Here's how the part is built. I have some questions about the finished solid (model axes, mm). Give positions to 0.01 mm unless a question says otherwise; leave off trailing zeros. Loops run counter-clockwise (first coordinate to the right, second up) from the corner with the lowest first, then second, coordinate; pieces in that order, holes last.
Q1. I need wall thicknesses on line 1 (Z direction, x = -27.5, y = 53); line 2 (Z direction, x = -27.65, y = 38.5); line 3 (Y direction, x = -26.05, z = 37.75). Which ranges of each line are inside material? Lowest first, please.
Q2. If we section it at B-B (y = 37): Please give me the cut outline in (x, z).
Q3. If we section it at A-A (z = 36.5): Please give me the cut outline in (x, y).
Q4. If we section it at C-C (x = -26.85): Please give me the cut outline in (y, z).
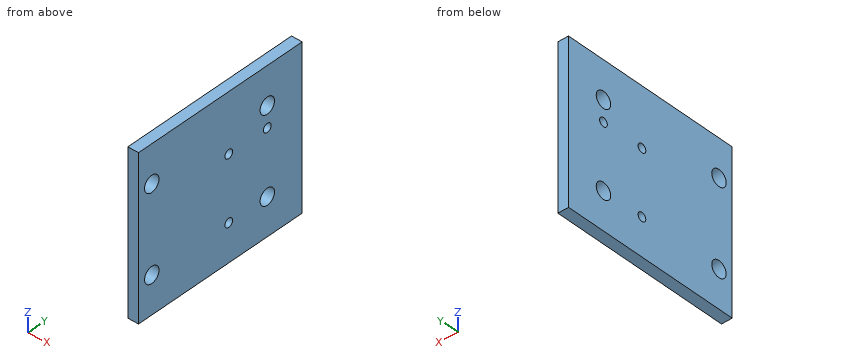
Autodesk Inventor part; units mm, degrees
ref_plane "YZ Plane" through (0, 0, 0) normal (1, 0, 0) x (0, 1, 0)
ref_plane "XZ Plane" through (0, 0, 0) normal (0, 1, 0) x (-1, 0, 0)
ref_plane "XY Plane" through (0, 0, 0) normal (0, 0, 1) x (1, 0, 0)
ref_plane "РабПлоскость1" through (-25.9085, 44.7403, 28.4958) normal (-1, 0, 0) x (0, 0, -1)
sketch "Эскиз1" plane through (-25.9085, 44.7403, 28.4958) normal (-1, 0, 0) x (0, 0, -1)
  line L0 (6, -10.75) -> (0, -10.75)
  line L1 (0, -10.75) -> (0, 48.15)
  line L2 (-14.95, -3.95) -> (14.95, -3.95)
  line L3 (14.95, -3.95) -> (14.95, -23.95)
  line L4 (14.95, -23.95) -> (-14.95, -23.95)
  line L5 (-14.95, -23.95) -> (-14.95, -3.95)
  line L6 (-14.95, -3.95) -> (14.95, -23.95) construction
  line L7 (14.95, -3.95) -> (-14.95, -23.95) construction
  point P0 (28.4958, 44.7403)
  point P1 (0, -13.95)
  dimension "d0" = 6
  dimension "d1" = 29.9
  dimension "d2" = 20
extrude "Выдавливание1" add sketch "Эскиз1" along normal blind 2
sketch "Эскиз2" plane through (-27.9085, 44.7403, 28.4958) normal (-1, 0, 0) x (0, 0, 1)
  line L0 (-14.95, 23.95) -> (-14.95, 3.95)
  line L1 (-14.95, 3.95) -> (14.95, 3.95)
  line L2 (14.95, 3.95) -> (14.95, -10.05)
  line L3 (14.95, -10.05) -> (-14.95, -10.05)
  line L4 (-14.95, -10.05) -> (-14.95, 3.95)
  point P0 (-28.4958, -44.7403)
  dimension "d5" = 14
extrude "Выдавливание2" add sketch "Эскиз2" against normal blind 2
sketch "Эскиз3" plane through (-27.9085, 44.7403, 28.4958) normal (-1, 0, 0) x (0, 0, 1)
  point P0 (-28.4958, -44.7403)
sketch "Эскиз4" plane through (-27.9085, 44.7403, 28.4958) normal (-1, 0, 0) x (0, 0, 1)
  circle A0 centre (-7.95, 16.7) radius 1.5
  circle A1 centre (-7.95, -7.3) radius 1.5
  circle A2 centre (7.95, -7.3) radius 1.5
  circle A3 centre (7.95, 16.7) radius 1.5
  point P0 (-28.4958, -44.7403)
extrude "Выдавливание3" cut sketch "Эскиз4" against normal blind 2
sketch "Эскиз5" plane through (-27.9085, 44.7403, 28.4958) normal (-1, 0, 0) x (0, 0, 1)
  circle A0 centre (4.05, 16.7) radius 0.8
  circle A1 centre (4.05, 8.7) radius 0.8
  circle A2 centre (-7.95, 8.7) radius 0.8
  circle A3 centre (-7.95, 16.7) radius 0.8
  point P0 (-28.4958, -44.7403)
extrude "Выдавливание4" cut sketch "Эскиз5" against normal blind 10 contours A0 | A1 | A2
properties part number "соединяет крепление с магнитом и рельсу"
Check sheet entries:
1. line 1: z = 13.55 to 19.88, 21.21 to 31.88, 33.21 to 43.45
1. line 2: z = 13.55 to 19.48, 21.61 to 35.38, 37.51 to 43.45
1. line 3: y = 34.69 to 36.7, 38.18 to 60.7, 62.18 to 68.69
2. outline: (-27.91, 13.55) - (-25.91, 13.55) - (-25.91, 19.11) - (-27.91, 19.11) - close; (-27.91, 21.98) - (-25.91, 21.98) - (-25.91, 35.01) - (-27.91, 35.01) - close; (-27.91, 37.88) - (-25.91, 37.88) - (-25.91, 43.45) - (-27.91, 43.45) - close
3. outline: (-27.91, 34.69) - (-25.91, 34.69) - (-25.91, 35.94) - (-27.91, 35.94) - close; (-27.91, 38.94) - (-25.91, 38.94) - (-25.91, 59.94) - (-27.91, 59.94) - close; (-27.91, 62.94) - (-25.91, 62.94) - (-25.91, 68.69) - (-27.91, 68.69) - close
4. outline: (34.69, 13.55) - (68.69, 13.55) - (68.69, 43.45) - (34.69, 43.45) - close; hole circle Ø3 at (37.44, 20.55); hole circle Ø3 at (37.44, 36.45); hole circle Ø1.6 at (53.44, 20.55); hole circle Ø1.6 at (53.44, 32.55); hole circle Ø3 at (61.44, 20.55); hole circle Ø3 at (61.44, 36.45); hole circle Ø1.6 at (61.44, 32.55)
